Part model, mm, in its own coordinate system. A direction names the side the tool comes from. Round coordinates to 2 decimals unless told otherwise and drop trailing zeros. Write each loop counter-clockwise with the first axis right and the second up, starting at its lowest first coordinate (ties: lowest second). Pieces come first, ordered by that corner, then holes.
```python
from build123d import *

# Parameters (mm, degrees)
F0_R     = 35
F1_DEPTH = 100
F2_R     = 10
F3_DEPTH = 40
F5_DEPTH = 20


with BuildPart() as f1:
    # F0 (on Right) → F1 (new body)
    with BuildSketch(Plane.YZ):
        Circle(F0_R)
    extrude(amount=F1_DEPTH)

    # F2 (on face) → F3 (join)
    with BuildSketch(Plane(origin=(0, 0, 0), x_dir=(0, -1, 0), z_dir=(-1, 0, 0))):
        Circle(F2_R)
    extrude(amount=F3_DEPTH)

    # F4 (on face) → F5 (join)
    with BuildSketch(Plane(origin=(-40, 0, 0), x_dir=(0, -1, 0), z_dir=(-1, 0, 0))):
        Polygon((-7.3776064835, -12.7783892676), (0, -25.5567785352), (7.3776064835, -12.7783892676), align=None)
        Polygon((-22.1328194504, -12.7783892676), (-7.3776064835, -12.7783892676), (-14.7552129669, 0), align=None)
        Polygon((-14.7552129669, 0), (-7.3776064835, -12.7783892676), (7.3776064835, -12.7783892676), (14.7552129669, 0), (7.3776064835, 12.7783892676), (-7.3776064835, 12.7783892676), align=None)
        Polygon((14.7552129669, 0), (7.3776064835, -12.7783892676), (22.1328194504, -12.7783892676), align=None)
        Polygon((-22.1328194504, 12.7783892676), (-14.7552129669, 0), (-7.3776064835, 12.7783892676), align=None)
        Polygon((7.3776064835, 12.7783892676), (14.7552129669, 0), (22.1328194504, 12.7783892676), align=None)
        Polygon((0, 25.5567785352), (-7.3776064835, 12.7783892676), (7.3776064835, 12.7783892676), align=None)
    extrude(amount=-F5_DEPTH)


solid = f1.part
```
Q1. Drop flat-ended pins along their axis: pin 1 (1.5 mm diameter, centred on x = 48, y = -9, fed in from -Z); pin 2 (1 mm diameter, centred on y = -19, z = 17, fed in from -X); pin 3 (12 mm diameter, centred on x = -27, y = -12, fed in from +Z). Give the stop position or say it passes through.
Values follow:
pin 1: stops at z = -34.01
pin 2: stops at x = 0
pin 3: stops at z = 15.16
Q2. Cut at C-C on x = -12. Write the cut outline in (y, z), plus the area to 3 significant figures.
Values follow:
outline: circle Ø20 at (0, 0)
area: 314 mm2
Q3. Cut at A-A on z = -17.5. Write the cut outline in (x, y).
Values follow:
outline: (-40, -4.65) - (-20, -4.65) - (-20, 4.65) - (-40, 4.65) - close; (0, -30.31) - (100, -30.31) - (100, 30.31) - (0, 30.31) - close
Q4. Mould opens along Z. For faces 1 (the flat face through (-30.14, 18.496, 6.479)), 2 (the flat face through (-30.14, 3.74, -19.08)), 3 (the flat face through (-30.14, -3.74, 19.08)) say: +Z half, -Z half, draft (parallel to the pull), parting line (faces both ways), or undercut.
Values follow:
face 1: undercut
face 2: -Z half
face 3: +Z half
Q5. Wall check: L1, parallel to X at y = 1, z = -15.5; L2, parallel to X at y = 19.5, z = 28.5; L3, parallel to Z at x = -32.5, y = -13. Give the ranges that are in metal, low to high.
Values follow:
L1: x = -40 to -20, 0 to 100
L2: x = 0 to 100
L3: z = -12.78 to 12.78
Q6. Cut at D-D on z = 2.5. Write the cut outline in (x, y), plus the area to 3 significant figures.
Values follow:
outline: (-40, -16.2) - (-20, -16.2) - (-20, -9.68) - (0, -9.68) - (0, -34.91) - (100, -34.91) - (100, 34.91) - (0, 34.91) - (0, 9.68) - (-20, 9.68) - (-20, 16.2) - (-40, 16.2) - close
area: 8,020 mm2
Q7. Cut at B-B on y = 19.5. Write the cut outline in (x, z), plus the area to 3 significant figures.
Values follow:
outline: (-40, -12.78) - (-20, -12.78) - (-20, -8.22) - (-40, -8.22) - close; (-40, 8.22) - (-20, 8.22) - (-20, 12.78) - (-40, 12.78) - close; (0, -29.06) - (100, -29.06) - (100, 29.06) - (0, 29.06) - close
area: 6,000 mm2
Q8. Which spindle directions (+Z, -Z, +X, -X, +Y, -Y) get a long thin tool onto all of the face, cutting with end or side? Do faces 4 (the flat face through (-30, -15, 12.778)), 5 (the flat face through (-20, 10.15, 0.36)), 6 (the flat face through (-30, 15, -12.778)), 7 (the flat face through (-30.14, 18.392, -6.3)). Say none if no direction does.
Values follow:
face 4: +Z, -X, -Y
face 5: none
face 6: -Z, -X, +Y
face 7: -X, +Y
